Here's the drawing with two shaded views (mm, measured from the low corner). I have some questions. A direction names the side the tool comes from. Give positions to 0.01 mm unless a question says otherwise; leave off trailing zeros. Loops run counter-clockwise (first coordinate to the right, second up) from the corner with the lowest first, then second, coordinate; pieces in that order, holes last. Notation, with made-up numbers: M 18,17.25 L 24,17.25 A17 ccw 24,24.25 Z; hole C 78,-13.75 d6. An arc over 180 degrees is marked long. Use CSV: the item, a comma, the result in double quotes.
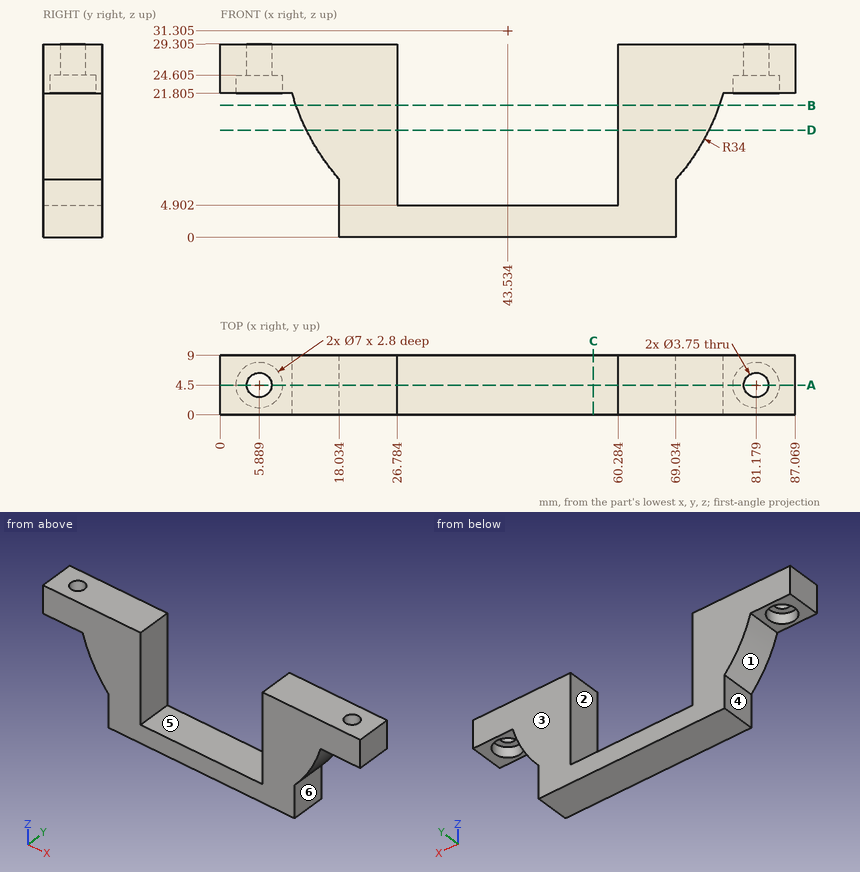
1. I'm going to push flat-ended pins straight in: pin 1 Ø3 at (y, z) = (8, 8) entering from -X; pin 2 Ø2.5 at (x, y) = (3.5, 4.5) entering from -Z (1 decimal); pin 3 Ø2 at (y, z) = (1, 10) entering from +X (1 decimal). Where does each tip first touch, or does it pass through?
Outcome:
pin 1,"x = 17.45"
pin 2,"z = 21.8"
pin 3,"x = 70.8"
2. I want a section at A-A, the plane y = 4.5. Give the number of separate pieces and of enclosed holes in the cut face, then the cut area to 3 significant figures.
Outcome:
separate pieces,"3"
enclosed holes,"0"
area,"982 mm2"
3. Which directions (+Z, -Z, +X, -X, +Y, -Y) give clear straight access to the entire face, cutting with the end or side of a thin tool? Please do the marked faces 4, 5 and 6.
Outcome:
face 4,"-Z, -X, +Y, -Y"
face 5,"+Z, +Y, -Y"
face 6,"-Z, +X, +Y, -Y"
4. I want a section at D-D, the plane z = 16.25. List the corners of the cut face in (x, y) for me (1 decimal), then the cut area to 3 significant figures.
Outcome:
outline,"M 13,0 L 26.8,0 L 26.8,9 L 13,9 Z; M 60.3,0 L 74,0 L 74,9 L 60.3,9 Z"
area,"247 mm2"
5. If we mould it in two halves opening along X, with no side actions, what happens to the marked faces 1, 2 and 3? For each: +X half, -X half, draft (parallel to the pull), parting line (faces both ways), or undercut.
Outcome:
face 1,"-X half"
face 2,"undercut"
face 3,"draft"
6. I want a section at C-C, the plane x = 56.5. List the corners of the cut face in (y, z) for me.
Outcome:
outline,"M 0,0 L 9,0 L 9,4.9 L 0,4.9 Z"
7. I want a section at B-B, the plane z = 20. List the corners of the cut face in (x, y) for me (1 decimal).
Outcome:
outline,"M 11.5,0 L 26.8,0 L 26.8,9 L 11.5,9 Z; M 60.3,0 L 75.6,0 L 75.6,9 L 60.3,9 Z"
8. Please list where these lines run through material, in increasing order: line 1 (Z direction, x = 6, y = 7.75) (1 decimal); line 2 (Z direction, x = 31.5, y = 3); line 3 (X direction, y = 1.75, z = 22.5) (1 decimal).
Outcome:
line 1,"24.6 to 29.3"
line 2,"0 to 4.9"
line 3,"0 to 3.7, 8.1 to 26.8, 60.3 to 79, 83.3 to 87.1"
